Design review of the part built by this model. Coordinates are the model's own, in mm. A direction names the side the tool comes from. Coordinates: 2 decimals unless noted, no trailing zeros. Loops run counter-clockwise (first coordinate to the right, second up) from the corner with the lowest first, then second, coordinate; pieces in that order, holes last. Notation, with made-up numbers: (36, 29) -> (73, 29) arc R30 ccw to (73, 52) -> close; hole circle Ø3 at (62.25, 47.25). An arc over 180 degrees is marked (long way). One line per item, written item: value. Start each with the question number.
1. Add section D-D on y = 0. Write out the cut boundary in (x, z), plus the area to 3 significant figures.
2. Add section C-C on x = 0. Write out the cut boundary in (y, z).
3. Insertion check: pin 1 (1.8 mm diameter, centred on y = -21, z = -3, fed in from -X); pin 2 (2 mm diameter, centred on x = 8, z = -8, fed in from -Y); pin 3 (0.6 mm diameter, centred on y = 19.5, z = -7, fed in from -X). Each pin has a flat end and moves straight along its axis. Give the tip position at first contact, or say it passes through.
4. Add section A-A on z = 2.5. Write out the cut boundary in (x, y), plus the area to 3 significant figures.
5. Machinability: for faces 1 (the flat face through (9, -1, 2)), 2 (the cylindrical face through (-0.187, -31.498, -7.437)), 3 (the flat face through (0, -28, -6.5)), which of the approach directions +Z, -Z, +X, -X, +Y, -Y give a long, thin tool a straight path to every point of the face, cutting with its end or side? Answer none if there is none.
6. Draft analysis for pull direction X (two halves, no side actions). For faces 4 (the cylindrical face through (0, -26, -2)), 5 (the conical face through (-0.117, 20.867, -8.571)), 6 (the flat face through (-10, 19, -7)), 7 (the flat face through (0, -32, 2)), state which applies: pulls with the +X half, pulls with the -X half, needs draft (parallel to the pull), parting line crosses it, or undercut.
7. Add section B-B on y = 12. Write out the cut boundary in (x, z), plus the area to 3 significant figures.
8. For probe 1 along Y at (x, z) = (0, 4.7); probe 2 along X at (y, z) = (-2, 3.5); probe 3 along X at (y, z) = (12, 4.75), list the stretches that pass through material, from the lowest coordinate up.
Autodesk Fusion 360 part; units mm, degrees
sketch "Sketch1" plane through (0, 0, 0) normal (0, 0, 1) x (1, 0, 0)
  line L0 (0, 60.043) -> (0, -60.043) construction
  line L1 (-62.1045, 0) -> (62.1045, 0) construction
  circle A0 centre (0, -23) radius 4.5
  line L2 (-4.4973, -23.1562) -> (-6.1, 23)
  line L3 (4.4973, -23.1562) -> (6.1, 23)
  line L4 (-11, 23) -> (11, 23)
  line L5 (11, 23) -> (11, -32)
  line L6 (11, -32) -> (-11, -32)
  line L7 (-11, -32) -> (-11, 23)
  line L8 (-10, 23) -> (10, 23)
  line L9 (10, 23) -> (10, 16)
  line L10 (10, 16) -> (-10, 16)
  line L11 (-10, 16) -> (-10, 23)
  circle A1 centre (0, -23) radius 8.5
  line L12 (-8.5, -23) -> (-8.5, -18.5)
  line L13 (-8.5, -18.5) -> (8.5, -18.5)
  line L14 (8.5, -18.5) -> (8.5, -23)
  circle A2 centre (0, -23) radius 3
  line L15 (-3, -23) -> (-3, -18.5)
  line L16 (3, -23) -> (3, -18.5)
  arc A3 (5.8569, 16) -> (-5.8569, 16) centre (0, 14.6976) ccw
  circle A4 centre (0, 12) radius 3
  line L17 (9, 21) -> (9, -30)
  line L18 (9, -30) -> (-9, -30)
  line L19 (-9, -30) -> (-9, 21)
  line L20 (-9, 21) -> (9, 21)
  line L21 (8.5, -18.5) -> (9, -18.5)
  line L22 (-8.5, -18.5) -> (-9, -18.5)
  dimension "d1" = 9
  dimension "d2" = 23
  dimension "d3" = 12.2
  dimension "d4" = 6.1
  dimension "d5" = 46
  dimension "d7" = 22
  dimension "d8" = 55
  dimension "d9" = 11
  dimension "d10" = 20
  dimension "d11" = 7
  dimension "d12" = 10
  dimension "d13" = 17
  dimension "d14" = 6
  dimension "d21" = 6
  dimension "d24" = 6
  dimension "d25" = 12
  dimension "d29" = 2
extrude "Extrude1" add sketch "Sketch1" along normal blind 3.8 contours A0 A2 L15 L16 | A0 L2 L13 L15 | A0 L2 L3 A1 L13 L18 | A0 L3 L13 L16 | A1 L12 L13 | A1 L13 L14 | L2 L10 L19 L20 | L2 L3 A3 L20 | A1 L12 L18 L19 L22 | L3 L10 L17 L20 | A1 L14 L17 L18 L21 | L2 L4 L8 L10 L11 L19 L20 | L2 L3 L4 L8 L20 | L4 L5 L6 L7 L9 L10 L11 A1 L17 L18 L19 | A1 L18 | L3 L4 L8 L9 L10 L17 L20 picked at (3.9634, -23.4711)
extrude "Extrude2" add sketch "Sketch1" against normal blind 6.5 contours A0 A2 L15 L16 | A0 L2 L13 L15 | A0 L3 L13 L16 | L2 L3 A3 L20 | L2 L3 L4 L8 L20 picked at (3.9634, -23.4711)
sketch "Sketch2" plane through (0, 0, -6.5) normal (0, 0, -1) x (1, 0, 0)
  line L0 (-5.8569, -16) -> (-6.1, -23)
  line L1 (-6.1, -23) -> (6.1, -23)
  line L2 (6.1, -23) -> (5.8569, -16)
  line L3 (10, -23) -> (10, -16)
  line L4 (10, -16) -> (-10, -16)
  line L5 (-10, -16) -> (-10, -23)
  line L6 (-10, -23) -> (10, -23)
  line L7 (-8.5, 18.5) -> (8.5, 18.5)
  line L8 (8.5, 18.5) -> (8.5, 23)
  circle A0 centre (0, 23) radius 8.5
  line L9 (-8.5, 23) -> (-8.5, 18.5)
  line L10 (-3, 18.5) -> (-3, 23)
  arc A1 (3, 23) -> (-3, 23) centre (0, 23) ccw
  line L11 (3, 23) -> (3, 18.5)
  line L12 (3, 18.5) -> (4.659, 18.5)
  line L13 (4.659, 18.5) -> (4.4973, 23.1562)
  arc A2 (4.4973, 23.1562) -> (-4.4973, 23.1562) centre (0, 23) ccw
  line L14 (-4.4973, 23.1562) -> (-4.659, 18.5)
  line L15 (-4.659, 18.5) -> (-3, 18.5)
  arc A3 (-5.8569, -16) -> (5.8569, -16) centre (0, -14.6976) ccw
  arc A4 (-5.8569, -16) -> (5.8569, -16) centre (0, -14.6976) ccw
extrude "Extrude3" add sketch "Sketch2" along normal blind 2.5 contours L0 L1 L2 L6 A3 A4 | L0 L4 L5 L6 | L2 L3 L4 L6 | L7 L10 A1 L11 L12 L13 A2 L14 L15 | L7 A0 L13 A2 L14 | L7 A0 L9 | L7 L8 A0
sketch "Sketch3" plane through (0, 0, 3.8) normal (0, 0, 1) x (-1, 0, 0)
  arc A0 (3, 23) -> (-3, 23) centre (0, 23) ccw
  line L0 (3, 23) -> (3, 18.5)
  line L1 (3, 18.5) -> (9, 18.5)
  arc A1 (-5.8569, -16) -> (5.8569, -16) centre (0, -14.6976) ccw
  line L2 (-9, 18.5) -> (-3, 18.5)
  line L3 (-3, 18.5) -> (-3, 23)
  line L4 (-11, -23) -> (11, -23)
  line L5 (11, -23) -> (11, 32)
  line L6 (11, 32) -> (-11, 32)
  line L7 (-11, 32) -> (-11, -23)
  line L8 (-11, -23) -> (11, -23)
  line L9 (11, -23) -> (11, 32)
  line L10 (-11, 32) -> (-11, -23)
  line L11 (11, 32) -> (-11, 32)
  line L12 (-9, -16) -> (-9, 18.5)
  line L13 (9, 18.5) -> (9, -16)
  line L14 (9, -16) -> (5.8569, -16)
  line L15 (-5.8569, -16) -> (-9, -16)
extrude "Extrude4" add sketch "Sketch3" along normal blind 2 contours A0 L0 L1 A1 L2 L3 L12 L13 L14 L15 | L4 L5 L6 L7 L8 L9 L10 L11
extrude "Extrude5" cut sketch "Sketch1" along normal blind 11 contours A4
sketch "Sketch4" plane through (0, 0, 5.8) normal (0, 0, 1) x (-1, 0, 0)
  circle A0 centre (0, -12) radius 3
  line L0 (11, 32) -> (-11, 32)
  line L1 (-11, 32) -> (-11, -23)
  line L2 (-11, -23) -> (11, -23)
  line L3 (11, -23) -> (11, 32)
  circle A1 centre (0, -12) radius 3
  circle A2 centre (0, -12) radius 4.6
  dimension "d30" = 9.2
  dimension "d39" = 22
extrude "Extrude6" cut sketch "Sketch4" against normal blind 0.5 contours A2
chamfer "Chamfer1" distance 1 angle 45 13 edges at (11, -4.5, 5.8) (-11, -4.5, 5.8) (0, -32, 5.8) (-11, -32, 2.9) (11, -32, 2.9) (3, -18.5, -2.6) (-3, -18.5, -2.6) (6.8295, -18.5, 0) (-6.8295, -18.5, 0) (-9, -1.25, 0) (9, -1.25, 0) (7.4285, 16, 0) (-7.4285, 16, 0)
chamfer "Chamfer1" distance 0.6 angle 45 2 faces at (-4.8333, -20, -9) (-8.4185, 18.8641, -9)
equation "d2 = ( 46 / 2 ) * 1 mm"
equation "d4 = d3 / 2"
equation "d5 = d2 * 2"
equation "d8 = d5 + 9 mm"
equation "d9 = d7 / 2"
equation "d12 = d10 / 2"
Worked answers:
1. outline: (-11, 0) -> (-10, 0) -> (-9, 1) -> (-9, 3.8) -> (9, 3.8) -> (9, 1) -> (10, 0) -> (11, 0) -> (11, 4.8) -> (10, 5.8) -> (-10, 5.8) -> (-11, 4.8) -> close
1. area: 57.2 mm²
2. outline: (-32, 0) -> (-27.5, 0) -> (-27.5, -6.5) -> (-31.5, -6.5) -> (-31.5, -8.4) -> (-30.9, -9) -> (-26.6, -9) -> (-26, -8.4) -> (-26, 3.8) -> (9, 3.8) -> (9, 5.3) -> (7.4, 5.3) -> (7.4, 5.8) -> (-31, 5.8) -> (-32, 4.8) -> close; (15, 3.8) -> (20.7, 3.8) -> (20.7, -8.4) -> (21.3, -9) -> (22.4, -9) -> (23, -8.4) -> (23, 5.8) -> (16.6, 5.8) -> (16.6, 5.3) -> (15, 5.3) -> close
3. pin 1: stops at x = -4.6
3. pin 2: stops at y = -27.82
3. pin 3: stops at x = -10
4. outline: (-11, -31) -> (-10, -32) -> (10, -32) -> (11, -31) -> (11, 23) -> (-11, 23) -> close; hole (-9, -18.5) -> (-4, -18.5) -> (-3, -19.5) -> (-3, -23) arc R3 ccw to (3, -23) -> (3, -19.5) -> (4, -18.5) -> (9, -18.5) -> (9, 16) -> (5.86, 16) arc R6 ccw to (-5.86, 16) -> (-9, 16) -> close
4. area: 505 mm²
5. face 1: -Z
5. face 2: -Z, -Y
5. face 3: -Y
6. face 4: undercut
6. face 5: undercut
6. face 6: pulls with the -X half
6. face 7: needs draft
7. outline: (-11, 0) -> (-10, 0) -> (-9, 1) -> (-9, 3.8) -> (-3, 3.8) -> (-3, 5.3) -> (-4.6, 5.3) -> (-4.6, 5.8) -> (-10, 5.8) -> (-11, 4.8) -> close; (3, 3.8) -> (9, 3.8) -> (9, 1) -> (10, 0) -> (11, 0) -> (11, 4.8) -> (10, 5.8) -> (4.6, 5.8) -> (4.6, 5.3) -> (3, 5.3) -> close
7. area: 43.6 mm²
8. probe 1: y = -32 to 9, 15 to 23
8. probe 2: x = -11 to -9, 9 to 11
8. probe 3: x = -11 to -3, 3 to 11
